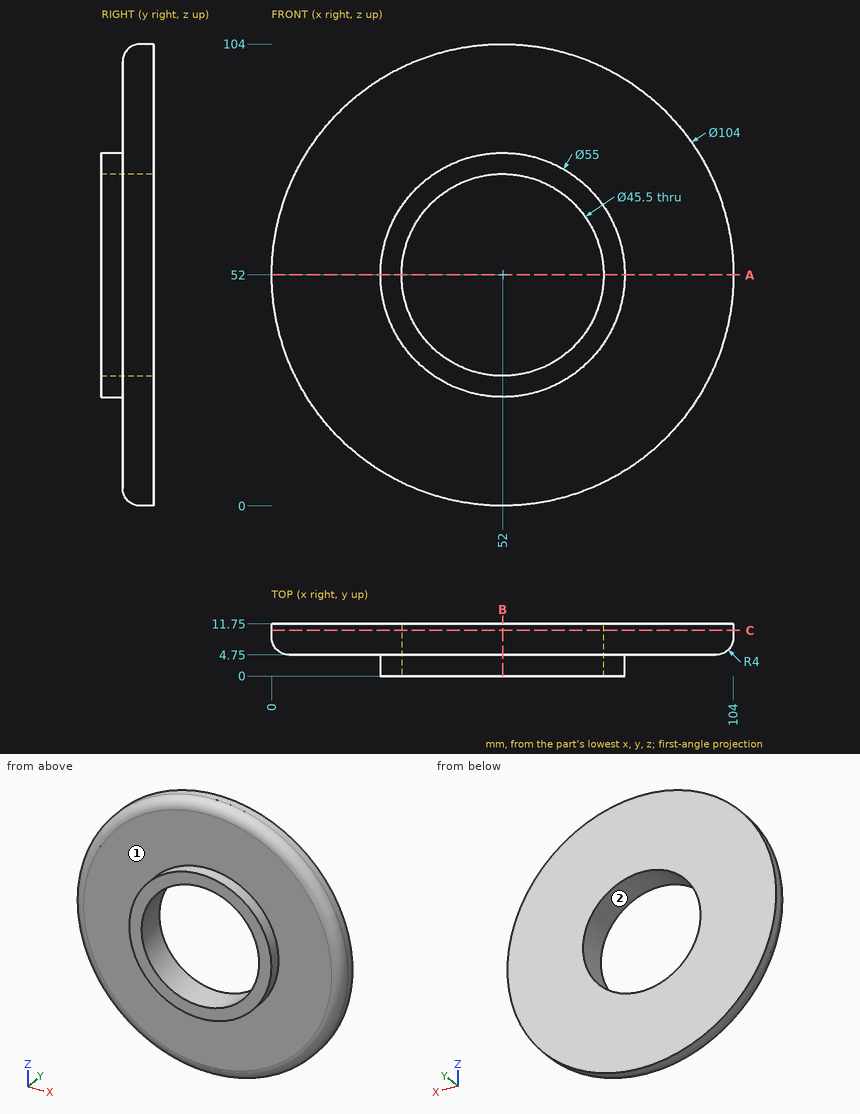
Design review of the part shown in the three views and the two pictorial views. Dimensions are in mm from the part's minimum x, y and z. A direction names the side the tool comes from. Give positions to 0.01 mm unless a question says otherwise; leave off trailing zeros. Order: outer loops, then holes, each group sorted by start corner. A loop starts at its lowest first (then second) coordinate and runs counter-clockwise, first axis right, second up. Notation, with made-up numbers: M 16,70 L 59,70 A30 ccw 59,94 Z; hole C 12.25,66 d3. An arc over 180 degrees is marked long. Answer in a Markdown table with one row per item. Add a question column.
(1) Consider section A-A on z = 52. State the section outline as (x, y) points, and give its area (3 significant figures).
(2) Consider section C-C on y = 10.25. State the section outline as (x, z) points.
(3) Consider section B-B on x = 52. State the section outline as (y, z) points.
(4) Wall thickness on probe 1 along Z at (x, y) = (52, 3); probe 2 along Y at (x, z) = (48, 90.5); probe 3 along Z at (x, y) = (36.5, 9.75): over which ranges is each line inside the solid? List them lowest first. Write a range as [from, to].
(5) For the marked faces 1 and 2, list the 3-axis set-ups (+Z, -Z, +X, -X, +Y, -Y) from which the entire face can be reached by the end or side of a thin tool; tool diameter is ignored.
(6) For pin 1 (6 mm diameter, centred on y = 1.5, z = 29, fed in from -X); pin 2 (2 mm diameter, centred on x = 65, y = 8.5, fed in from -Z); pin 3 (5 mm diameter, centred on x = 71.5, z = 19, fed in from -Y), all flat-tipped, find the tip position at first contact; note any pin that passes through.
Evaluation:
| question | item | result |
|---|---|---|
| 1 | outline | M 0,8.75 A4 ccw 4,4.75 L 24.5,4.75 L 24.5,0 L 29.25,0 L 29.25,11.75 L 0,11.75 Z; M 74.75,0 L 79.5,0 L 79.5,4.75 L 100,4.75 A4 ccw 104,8.75 L 104,11.75 L 74.75,11.75 Z |
| 1 | area | 448 mm^2 |
| 2 | outline | C 52,52 d104; hole C 52,52 d45.5 |
| 3 | outline | M 0,24.5 L 4.75,24.5 L 4.75,4 A4 ccw 8.75,0 L 11.75,0 L 11.75,29.25 L 0,29.25 Z; M 0,74.75 L 11.75,74.75 L 11.75,104 L 8.75,104 A4 ccw 4.75,100 L 4.75,79.5 L 0,79.5 Z |
| 4 | probe 1 | z = [24.5, 29.25], [74.75, 79.5] |
| 4 | probe 2 | y = [4.75, 11.75] |
| 4 | probe 3 | z = [2.36, 35.35], [68.65, 101.64] |
| 5 | face 1 | -Y |
| 5 | face 2 | +Y, -Y |
| 6 | pin 1 | stops at x = 33.13 |
| 6 | pin 2 | stops at z = 1.41 |
| 6 | pin 3 | stops at y = 4.75 |
